from build123d import *

# Parameters (mm, degrees)
ESQUISSE1_W                  = 198
ESQUISSE1_H                  = 320
BOSS_EXTRU_1_DEPTH           = 3
ENL_V_MAT_EXTRU_1_REACH      = 194.445
ESQUISSE2_R                  = 2.2
ENL_V_MAT_EXTRU_4_REACH      = 194.445
ESQUISSE5_W                  = 20
ESQUISSE5_H                  = 20
ENL_V_MAT_EXTRU_5_DEPTH      = 193.44479728
ENL_V_MAT_EXTRU_5_DEPTH_BACK = 193.44479728
ESQUISSE7_W                  = 37
ESQUISSE7_H                  = 20
ESQUISSE7_W_2                = 16
CONG_2_R                     = 3
ENL_V_MAT_EXTRU_6_REACH      = 194.445


with BuildPart() as part:
    # Esquisse1 → Boss.-Extru.1 (new body)
    with BuildSketch(Plane.XY):
        with Locations((0, 5)):
            Rectangle(ESQUISSE1_W, ESQUISSE1_H)
    extrude(amount=BOSS_EXTRU_1_DEPTH)

    # Esquisse2 → Enlèv. mat.-Extru.1 (cut, up to next)
    with BuildSketch(Plane.XY.offset(3), mode=Mode.PRIVATE) as enl_v_mat_extru_1_sk1:
        with Locations((9, -145)):
            Circle(ESQUISSE2_R)
    enl_v_mat_extru_1_tool1 = extrude(enl_v_mat_extru_1_sk1.sketch, amount=-ENL_V_MAT_EXTRU_1_REACH, mode=Mode.PRIVATE) & part.part
    # Esquisse2 → Enlèv. mat.-Extru.1 (cut, up to next)
    with BuildSketch(Plane.XY.offset(3), mode=Mode.PRIVATE) as enl_v_mat_extru_1_sk2:
        with Locations((-9, -145)):
            Circle(ESQUISSE2_R)
    enl_v_mat_extru_1_tool2 = extrude(enl_v_mat_extru_1_sk2.sketch, amount=-ENL_V_MAT_EXTRU_1_REACH, mode=Mode.PRIVATE) & part.part
    # Esquisse2 → Enlèv. mat.-Extru.1 (cut, up to next)
    with BuildSketch(Plane.XY.offset(3), mode=Mode.PRIVATE) as enl_v_mat_extru_1_sk3:
        with Locations((-9, 155)):
            Circle(ESQUISSE2_R)
    enl_v_mat_extru_1_tool3 = extrude(enl_v_mat_extru_1_sk3.sketch, amount=-ENL_V_MAT_EXTRU_1_REACH, mode=Mode.PRIVATE) & part.part
    # Esquisse2 → Enlèv. mat.-Extru.1 (cut, up to next)
    with BuildSketch(Plane.XY.offset(3), mode=Mode.PRIVATE) as enl_v_mat_extru_1_sk4:
        with Locations((9, 155)):
            Circle(ESQUISSE2_R)
    enl_v_mat_extru_1_tool4 = extrude(enl_v_mat_extru_1_sk4.sketch, amount=-ENL_V_MAT_EXTRU_1_REACH, mode=Mode.PRIVATE) & part.part
    add(enl_v_mat_extru_1_tool1.solids().sort_by_distance((9, -145, 3))[0], mode=Mode.SUBTRACT)
    add(enl_v_mat_extru_1_tool2.solids().sort_by_distance((-9, -145, 3))[0], mode=Mode.SUBTRACT)
    add(enl_v_mat_extru_1_tool3.solids().sort_by_distance((-9, 155, 3))[0], mode=Mode.SUBTRACT)
    add(enl_v_mat_extru_1_tool4.solids().sort_by_distance((9, 155, 3))[0], mode=Mode.SUBTRACT)

    # Esquisse5 → Enlèv. mat.-Extru.4 (cut, up to next)
    with BuildSketch(Plane.XY.offset(3), mode=Mode.PRIVATE) as enl_v_mat_extru_4_sk1:
        with Locations((-68.5, 88)):
            Rectangle(ESQUISSE5_W, ESQUISSE5_H)
    enl_v_mat_extru_4_tool1 = extrude(enl_v_mat_extru_4_sk1.sketch, amount=-ENL_V_MAT_EXTRU_4_REACH, mode=Mode.PRIVATE) & part.part
    # Esquisse5 → Enlèv. mat.-Extru.4 (cut, up to next)
    with BuildSketch(Plane.XY.offset(3), mode=Mode.PRIVATE) as enl_v_mat_extru_4_sk2:
        with Locations((-11.5, 88)):
            Rectangle(ESQUISSE5_W, ESQUISSE5_H)
    enl_v_mat_extru_4_tool2 = extrude(enl_v_mat_extru_4_sk2.sketch, amount=-ENL_V_MAT_EXTRU_4_REACH, mode=Mode.PRIVATE) & part.part
    # Esquisse5 → Enlèv. mat.-Extru.4 (cut, up to next)
    with BuildSketch(Plane.XY.offset(3), mode=Mode.PRIVATE) as enl_v_mat_extru_4_sk3:
        with Locations((45.5, 88)):
            Rectangle(ESQUISSE5_W, ESQUISSE5_H)
    enl_v_mat_extru_4_tool3 = extrude(enl_v_mat_extru_4_sk3.sketch, amount=-ENL_V_MAT_EXTRU_4_REACH, mode=Mode.PRIVATE) & part.part
    add(enl_v_mat_extru_4_tool1.solids().sort_by_distance((-68.5, 88, 3))[0], mode=Mode.SUBTRACT)
    add(enl_v_mat_extru_4_tool2.solids().sort_by_distance((-11.5, 88, 3))[0], mode=Mode.SUBTRACT)
    add(enl_v_mat_extru_4_tool3.solids().sort_by_distance((45.5, 88, 3))[0], mode=Mode.SUBTRACT)

    # Esquisse7 → Enlèv. mat.-Extru.5 (cut, two sides: drawn at the far end of the back side and taken through both)
    with BuildSketch(Plane.XY.offset(3).offset(-ENL_V_MAT_EXTRU_5_DEPTH_BACK)):
        with Locations((-40, 88)):
            Rectangle(ESQUISSE7_W, ESQUISSE7_H)
        with Locations((17, 88)):
            Rectangle(ESQUISSE7_W, ESQUISSE7_H)
        with Locations((63.5, 88)):
            Rectangle(ESQUISSE7_W_2, ESQUISSE7_H)
    extrude(amount=ENL_V_MAT_EXTRU_5_DEPTH + ENL_V_MAT_EXTRU_5_DEPTH_BACK, mode=Mode.SUBTRACT)

    # Congé2
    cong_2_edges = [part.edges().sort_by_distance(p)[0] for p in [
        (-78.5, 78, 1.5),
        (-78.5, 98, 1.5),
        (71.5, 98, 1.5),
        (71.5, 78, 1.5),
    ]]
    fillet(cong_2_edges, radius=CONG_2_R)

    # Esquisse9 → Enlèv. mat.-Extru.6 (cut, up to next)
    with BuildSketch(Plane.XY.offset(3), mode=Mode.PRIVATE) as enl_v_mat_extru_6_sk1:
        Polygon((-3.5, 28), (13.5, 28), (22.5, 37), (22.5, 78), (-29.5, 78), (-29.5, 37), (-20.5, 28), align=None)
    enl_v_mat_extru_6_tool1 = extrude(enl_v_mat_extru_6_sk1.sketch, amount=-ENL_V_MAT_EXTRU_6_REACH, mode=Mode.PRIVATE) & part.part
    add(enl_v_mat_extru_6_tool1.solids().sort_by_distance((-3.5, 53.707424, 3))[0], mode=Mode.SUBTRACT)


solid = part.part
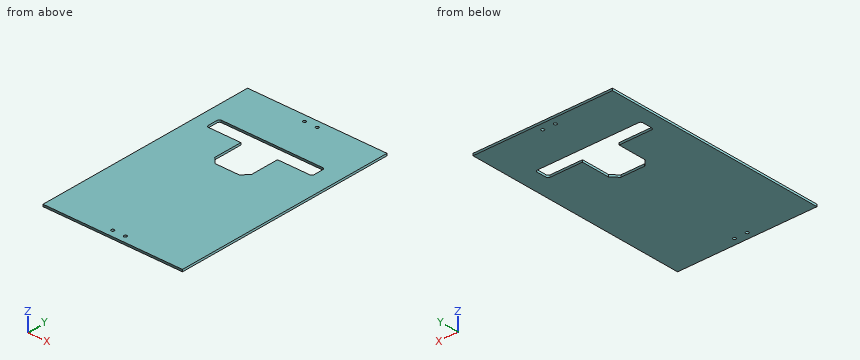
Check sheet for the modelled part. Datum: model origin and axes. Units: mm. Coordinates: 2 decimals unless noted, no trailing zeros. Write each loop counter-clockwise with the first axis right and the second up, starting at its lowest first coordinate (ties: lowest second). Pieces come first, ordered by that corner, then holes. Notation, with made-up numbers: M -7,10.5 L 6,10.5 A26 ccw 6,31.5 Z; hole C -21.75,59.25 d11. An arc over 180 degrees is marked long. Answer as CSV lines item,"result".
Q1. Cross-section at A-A (x = -39.5). Record the boundary of the cut face in (y, z), then the cut area to 3 significant figures.
Check result:
outline,"M -155,0 L 78,0 L 78,3 L -155,3 Z; M 98,0 L 165,0 L 165,3 L 98,3 Z"
area,"900 mm^2"
Q2. Cross-section at B-B (z = 0.9). Record the boundary of the cut face in (x, y).
Check result:
outline,"M -99,-155 L 99,-155 L 99,165 L -99,165 Z; hole M -78.5,81 A3 ccw -75.5,78 L -29.5,78 L -29.5,37 L -20.5,28 L 13.5,28 L 22.5,37 L 22.5,78 L 68.5,78 A3 ccw 71.5,81 L 71.5,95 A3 ccw 68.5,98 L -75.5,98 A3 ccw -78.5,95 Z; hole C -9,-145 d4.4; hole C -9,155 d4.4; hole C 9,-145 d4.4; hole C 9,155 d4.4"
Q3. Material ranges on probe 1 along X at (y, z) = (-145, 0.85); probe 2 along Y at (x, z) = (-9, 1.25); probe 3 along Y at (x, z) = (-61.5, 1.4), recorded low to high. Write a range as from..to.
Check result:
probe 1,"-99..-11.2, -6.8..6.8, 11.2..99"
probe 2,"-155..-147.2, -142.8..28, 98..152.8, 157.2..165"
probe 3,"-155..78, 98..165"
